Design review of the part built by this model. Coordinates are the model's own, in mm. A direction names the side the tool comes from. Round coordinates to 2 decimals unless told otherwise and drop trailing zeros. Order: outer loops, then holes, each group sorted by start corner. A loop starts at its lowest first (then second) coordinate and runs counter-clockwise, first axis right, second up. Notation, with made-up numbers: (13.25, -10.75) - (20.25, -10.75) arc R7 ccw to (20.25, -4.75) - close; hole circle Ø9 at (24.25, 23.25). An arc over 180 degrees is marked (long way). Use CSV: the item, a comma, the result in double quotes.
from build123d import *

# Parameters (mm, degrees)
SKETCH2_R           = 3
BOSS_EXTRUDE1_DEPTH = 13
BOSS_EXTRUDE2_DEPTH = 8
SKETCH6_R           = 3
SKETCH6_R_2         = 2.5
CUT_EXTRUDE1_DEPTH  = 1
CHAMFER1_SIZE       = 0.4
SKETCH7_R           = 0.2
CUT_EXTRUDE2_DEPTH  = 14


with BuildPart() as part:
    # Sketch2 → Boss-Extrude1 (new body)
    with BuildSketch(Plane(origin=(0, 0, 0), x_dir=(1, 0, 0), z_dir=(0, 1, 0))):
        Circle(SKETCH2_R)
    extrude(amount=BOSS_EXTRUDE1_DEPTH)

    # Sketch3 → Boss-Extrude2 (add)
    with BuildSketch(Plane.XZ):
        Polygon((1.732050808, -3), (3.464101615, 0), (1.732050808, 3), (-1.732050808, 3), (-3.464101615, 0), (-1.732050808, -3), align=None)
    extrude(amount=-BOSS_EXTRUDE2_DEPTH)

    # Sketch4 → Cut-Revolve3 (revolve, cut)
    with BuildSketch(Plane.XY):
        Polygon((-0.45, 0), (-3.464101615, 4), (-3.464101615, 0), align=None)
    revolve(axis=Axis((0, 0, 0), (0, 1, 0)), mode=Mode.SUBTRACT)

    # Sketch6 → Cut-Extrude1 (cut)
    with BuildSketch(Plane(origin=(0, 8, 0), x_dir=(1, 0, 0), z_dir=(0, 1, 0))):
        Circle(SKETCH6_R)
        Circle(SKETCH6_R_2, mode=Mode.SUBTRACT)
    extrude(amount=CUT_EXTRUDE1_DEPTH, mode=Mode.SUBTRACT)

    # Chamfer1
    chamfer1_edges = [part.edges().sort_by_distance(p)[0] for p in [
        (-3, 13, 0),
    ]]
    chamfer(chamfer1_edges, length=CHAMFER1_SIZE)

    # Sketch7 → Cut-Extrude2 (cut, through all)
    with BuildSketch(Plane.XZ):
        Circle(SKETCH7_R)
    extrude(amount=-CUT_EXTRUDE2_DEPTH, mode=Mode.SUBTRACT)

    # Sketch9 → CBORE for #0 Fillister Head Machine Screw1 (revolve, cut)
    with BuildSketch(Plane(origin=(0, 13, 0), x_dir=(0, 0, 1), z_dir=(1, 0, 0))):
        Polygon((0, 0), (0, 13), (0.889, 13), (0.889, 1.397), (1.38938, 1.397), (1.38938, 0.635), (2.02438, 0), align=None)
    revolve(axis=Axis((0, 19.35, 0), (0, -1, 0)), mode=Mode.SUBTRACT)


solid = part.part
1) Insertion check: pin 1 Ø3 at (x, z) = (0, 0.5) entering from +Y. The pin has a flat end and moves straight along its axis. Give the tip position at first contact, or say it passes through.
Data:
pin 1,"stops at y = 12.98"
2) We need section B-B (x = 0). Give the boundary of the cut face in (y, z) (3 decimals), then the cut area to 3 significant figures.
Data:
outline,"(0.583, -0.889) - (3.384, -3) - (8, -3) - (8, -2.5) - (9, -2.5) - (9, -3) - (12.6, -3) - (13, -2.6) - (13, -2.024) - (12.365, -1.389) - (11.603, -1.389) - (11.603, -0.889) - close; (0.583, 0.889) - (11.603, 0.889) - (11.603, 1.389) - (12.365, 1.389) - (13, 2.024) - (13, 2.6) - (12.6, 3) - (9, 3) - (9, 2.5) - (8, 2.5) - (8, 3) - (3.384, 3) - close"
area,"43.6 mm2"
3) The part is to be moulded in two halves that separate along Z. For faces 4 (the face through (0.87, 6.17, -0.19)), 5 (the face through (1.356, 11.989, -0.301)), 6 (the face through (-2.6, 5.7, 1.5)), 7 (the face through (-0.54, 8.49, 2.44)), say which applies: +Z half, -Z half, draft (parallel to the pull), parting line (faces both ways), or undercut.
Data:
face 4,"undercut"
face 5,"undercut"
face 6,"+Z half"
face 7,"parting line"
4) We need section C-C (y = 11.25). Give the boundary of the cut face in (x, z), then the cut area to 3 significant figures.
Data:
outline,"circle Ø6 at (0, 0); hole circle Ø1.78 at (0, 0)"
area,"25.8 mm2"
5) To check wall thickness, follow L1, parallel to Z at x = 0, y = 11.8; L2, parallel to X at y = 8.75, z = 0. State the ranges of each line that lie inside material, in increasing order. Write a range as from..to.
Data:
L1,"z = -3..-1.39, 1.39..3"
L2,"x = -2.5..-0.89, 0.89..2.5"
6) We need section A-A (y = 4.5). Give the boundary of the cut face in (x, z).
Data:
outline,"(-3.46, 0) - (-1.73, -3) - (1.73, -3) - (3.46, 0) - (1.73, 3) - (-1.73, 3) - close; hole circle Ø1.78 at (0, 0)"
7) For faces 1 (the face through (-3, 11, 0)), 2 (the face through (3, 8, 0)), 3 (the face through (2.6, 5.7, 1.5)), list the 3-axis set-ups (+Z, -Z, +X, -X, +Y, -Y) from which the entire face can be reached by the end or side of a thin tool; tool diameter is ignored.
Data:
face 1,"+Y"
face 2,"none"
face 3,"+Z, +X, +Y, -Y"
